```python
from build123d import *

# Parameters (mm, degrees)
SKETCH1_R           = 5
BOSS_EXTRUDE1_DEPTH = 10
FILLET1_R           = 2.54
SCALE1_SCALE        = 0.66


with BuildPart() as part:
    # Sketch1 → Boss-Extrude1 (new body)
    with BuildSketch(Plane(origin=(0, 0, 0), x_dir=(1, 0, 0), z_dir=(0, 1, 0))):
        with BuildLine():
            Line((-6.590776184, -6.25), (43.090776184, -6.25))
            ThreePointArc((43.090776184, -6.25), (46.152638362, -6.730283618), (48.920388092, -8.125))
            ThreePointArc((48.920388092, -8.125), (64.75, 0), (48.920388092, 8.125))
            ThreePointArc((48.920388092, 8.125), (46.152638362, 6.730283618), (43.090776184, 6.25))
            Line((43.090776184, 6.25), (-6.590776184, 6.25))
            ThreePointArc((-6.590776184, 6.25), (-9.652638362, 6.730283618), (-12.420388092, 8.125))
            ThreePointArc((-12.420388092, 8.125), (-28.25, 0), (-12.420388092, -8.125))
            ThreePointArc((-12.420388092, -8.125), (-9.652638362, -6.730283618), (-6.590776184, -6.25))
        make_face()
        with Locations((-18.25, 0)):
            Circle(SKETCH1_R, mode=Mode.SUBTRACT)
        with Locations((54.75, 0)):
            Circle(SKETCH1_R, mode=Mode.SUBTRACT)
    extrude(amount=BOSS_EXTRUDE1_DEPTH)

    # Fillet1
    fillet1_edges = [part.edges().sort_by_distance(p)[0] for p in [
        (-9.652638362, 10, 6.730283618),
        (-28.25, 0, 0),
        (-9.652638362, 0, -6.730283618),
        (18.25, 10, 6.25),
        (46.152638362, 10, 6.730283618),
        (64.75, 10, 0),
        (46.152638362, 10, -6.730283618),
        (18.25, 10, -6.25),
        (-9.652638362, 10, -6.730283618),
        (-28.25, 10, 0),
        (18.25, 0, -6.25),
        (46.152638362, 0, -6.730283618),
        (64.75, 0, 0),
        (46.152638362, 0, 6.730283618),
        (18.25, 0, 6.25),
        (-9.652638362, 0, 6.730283618),
    ]]
    fillet(fillet1_edges, radius=FILLET1_R)


with BuildPart() as part_1:
    # Scale1: scaled about (18.25, 5, 0)
    add(part.part.scale(SCALE1_SCALE).moved(Location((6.205, 1.7, 0))))


solid = part_1.part
```
For this review, take the finished solid that the model builds, in its own axes (mm). A direction names the side the tool comes from. Round coordinates to 2 decimals unless told otherwise and drop trailing zeros. Write each loop counter-clockwise with the first axis right and the second up, starting at its lowest first coordinate (ties: lowest second). Pieces come first, ordered by that corner, then holes. Notation, with made-up numbers: (-9.5, 63.5) - (32.5, 63.5) arc R27 ccw to (32.5, 95.5) - close; hole circle Ø11 at (13.25, 53.5). An arc over 180 degrees is marked (long way). Answer as a JSON object with one key per item and string values.
1. We need section D-D on y = 2.25. Give the boundary of the cut face in (x, z) (3 decimals), then the cut area to 3 significant figures.
Response values:
{"outline": "(-2.246, -5.009) arc R7.035 cw to (1.855, -3.69) - (34.645, -3.69) arc R7.035 cw to (38.746, -5.009) arc R6.165 ccw (long way) to (38.746, 5.009) arc R7.035 cw to (34.645, 3.69) - (1.855, 3.69) arc R7.035 cw to (-2.246, 5.009) arc R6.165 ccw (long way) to start; hole circle Ø6.6 at (-5.84, 0); hole circle Ø6.6 at (42.34, 0)", "area": "444 mm2"}
2. We need section C-C on x = 22. Give the boundary of the cut face in (y, z) (3 decimals).
Response values:
{"outline": "(1.7, -2.449) arc R1.676 ccw to (3.376, -4.125) - (6.624, -4.125) arc R1.676 ccw to (8.3, -2.449) - (8.3, 2.449) arc R1.676 ccw to (6.624, 4.125) - (3.376, 4.125) arc R1.676 ccw to (1.7, 2.449) - close"}
3. We need section B-B on y = 4.75. Give the boundary of the cut face in (x, z) (1 decimal).
Response values:
{"outline": "(-2, -5.4) arc R6.6 cw to (1.9, -4.1) - (34.6, -4.1) arc R6.6 cw to (38.5, -5.4) arc R6.6 ccw (long way) to (38.5, 5.4) arc R6.6 cw to (34.6, 4.1) - (1.9, 4.1) arc R6.6 cw to (-2, 5.4) arc R6.6 ccw (long way) to start; hole circle Ø6.6 at (-5.8, 0); hole circle Ø6.6 at (42.3, 0)"}
4. Tool access review of faces 3 (the face through (18.02, 2.204, -3.647)), 4 (the face through (18.48, 2.204, 3.647)), 5 (the face through (18, 5, 4.125)), 6 (the face through (18.48, 7.796, 3.647)), 7 (the face through (18, 5, -4.125)): name each direction out of +Z, -Z, +X, -X, +Y, -Y from which nothing blocks a thin tool from reaching the whole face with its end or side.
Response values:
{"face 3": "-Z, -Y", "face 4": "+Z, -Y", "face 5": "+Z, +Y, -Y", "face 6": "+Z, +Y", "face 7": "-Z, +Y, -Y"}
5. We need section A-A on z = 0. Give the boundary of the cut face in (x, y).
Response values:
{"outline": "(-12.44, 3.38) arc R1.68 ccw to (-10.76, 1.7) - (-9.14, 1.7) - (-9.14, 8.3) - (-10.76, 8.3) arc R1.68 ccw to (-12.44, 6.62) - close; (-2.54, 1.7) - (39.04, 1.7) - (39.04, 8.3) - (-2.54, 8.3) - close; (45.64, 1.7) - (47.26, 1.7) arc R1.68 ccw to (48.94, 3.38) - (48.94, 6.62) arc R1.68 ccw to (47.26, 8.3) - (45.64, 8.3) - close"}
6. For pin 1 Ø3.5 at (x, y) = (19, 4.5) entering from -Z (3 decimals); pin 2 Ø2 at (x, z) = (32, -4) entering from +Y; pin 3 Ø2.5 at (x, y) = (11.5, 4.5) entering from +Z (3 decimals), all flat-tipped, find the tip position at first contact; note any pin that passes through.
Response values:
{"pin 1": "stops at z = -4.125", "pin 2": "stops at y = 8.21", "pin 3": "stops at z = 4.125"}
7. To check wall thickness, follow line 1 along X through (y, z) = (3.25, 0); line 2 along Z through (x, y) = (-5.84, 5.5); line 3 along X through (y, z) = (2.5, 0.75). State the ranges of each line that lie inside material, in increasing order.
Response values:
{"line 1": "x = -12.44 to -9.14, -2.54 to 39.04, 45.64 to 48.94", "line 2": "z = -6.6 to -3.3, 3.3 to 6.6", "line 3": "x = -12.15 to -9.05, -2.63 to 39.13, 45.55 to 48.65"}
8. Draft analysis for pull direction X (two halves, no side actions). For faces 1 (the face through (45.49, 4.95, -0.99)), 2 (the face through (18, 1.7, 0)), state which applies: +X half, -X half, draft (parallel to the pull), parting line (faces both ways), or undercut.
Response values:
{"face 1": "undercut", "face 2": "draft"}
